For this review, take the finished solid that the model builds, in its own axes (mm). Give positions to 0.01 mm unless a question says otherwise; leave off trailing zeros. Loops run counter-clockwise (first coordinate to the right, second up) from the corner with the lowest first, then second, coordinate; pieces in that order, holes last. Notation, with made-up numbers: (36, -9) -> (88, -9) arc R24 cw to (88, 14) -> close; hole circle Ø3 at (33, -22). An arc over 180 degrees is marked (long way). One line per question, with ' | ' between items. Start each with the question number.
(1) Insertion check: P1, Ø1.2, axis at x = 77, y = 9, coming from the +Z side; P2, Ø1.2, axis at x = 81, y = 1.5, coming from the -Z side; P3, Ø1.5, axis at x = 176.5, z = -41, coming from the -Y side. Each pin has a flat end and moves straight along its axis. Give the tip position at first contact, or say it passes through.
(2) Wall thickness on probe 1 along Z at (x, y) = (120, 1.25): over which ranges is the line inside the solid? List them lowest first.
(3) Consider section A-A (x = 66.5). Write out the cut boundary in (y, z).
Autodesk Inventor part; units mm, degrees
ref_plane "YZ Plane" through (0, 0, 0) normal (1, 0, 0) x (0, 1, 0)
ref_plane "XZ Plane" through (0, 0, 0) normal (0, 1, 0) x (-1, 0, 0)
ref_plane "XY Plane" through (0, 0, 0) normal (0, 0, 1) x (1, 0, 0)
sketch "Skizze2" plane through (0, 0, 0) normal (0, 1, 0) x (-1, 0, 0)
  line L0 (27.6477, 247.101) -> (-272.3523, 247.101)
  line L1 (-272.3523, 247.101) -> (-272.3523, -42.899)
  line L2 (-272.3523, -42.899) -> (27.6477, -42.899)
  line L3 (27.6477, -42.899) -> (27.6477, 247.101)
  point P0 (0, 0)
  dimension "d1" = 290
  dimension "d2" = 300
extrude "Extrusion1" add sketch "Skizze2" along normal blind 10
sketch "Skizze3" plane through (-27.6477, 0, 247.101) normal (0, 0, 1) x (1, 0, 0)
  point P0 (27.6477, 0)
sketch "Skizze4" plane through (-27.6477, 0, 247.101) normal (0, 0, 1) x (1, 0, 0)
  line L0 (0, 10) -> (300, 10)
  line L1 (0, 0) -> (0, 10)
  line L2 (300, 0) -> (300, 10)
  line L3 (0, 7.5) -> (300, 7.5)
  line L4 (300, 7.5) -> (300, 2.5)
  line L5 (300, 2.5) -> (0, 2.5)
  line L6 (0, 2.5) -> (0, 7.5)
  line L7 (0, 0) -> (300, 0)
  line L8 (0, 10) -> (300, 10)
  line L9 (300, 10) -> (300, 0)
  line L10 (300, 0) -> (0, 0)
  line L11 (0, 0) -> (0, 10)
  dimension "d8" = 2.5
  dimension "d9" = 2.5
extrude "Extrusion2" cut sketch "Skizze4" against normal blind 5 contours L0 L2 L3 L1 | L5 L2 L7 L1
sketch "Skizze5" plane through (272.3523, 0, -42.899) normal (0, 0, -1) x (-1, 0, 0)
  line L0 (0, 0) -> (0, 10)
  line L1 (0, 7.5) -> (300, 7.5)
  line L2 (300, 7.5) -> (300, 2.5)
  line L3 (300, 2.5) -> (0, 2.5)
  line L4 (0, 2.5) -> (0, 7.5)
  line L5 (0, 10) -> (300, 10)
  line L6 (0, 0) -> (300, 0)
  line L7 (300, 10) -> (0, 10)
  line L8 (300, 10) -> (0, 10)
  line L9 (0, 10) -> (0, 0)
  line L10 (0, 0) -> (300, 0)
  line L11 (300, 0) -> (300, 10)
  point P0 (272.3523, 0)
  dimension "d12" = 2.5
  dimension "d13" = 2.5
extrude "Extrusion3" cut sketch "Skizze5" against normal blind 5 contours L0 L3 L11 L6 | L0 L5 L11 L1
properties material "Holz (Ahorn)"
A:
1) P1: stops at z = 242.1 | P2: stops at z = -37.9 | P3: stops at y = 2.5
2) probe 1: z = -37.9 to 242.1
3) outline: (0, -37.9) -> (2.5, -37.9) -> (2.5, -42.9) -> (7.5, -42.9) -> (7.5, -37.9) -> (10, -37.9) -> (10, 242.1) -> (7.5, 242.1) -> (7.5, 247.1) -> (2.5, 247.1) -> (2.5, 242.1) -> (0, 242.1) -> close
